Check sheet for the modelled part. Datum: model origin and axes. Units: mm. Face numbers are marked on the shaded views. A direction names the side the tool comes from. Give positions to 0.01 mm unless a question says otherwise; leave off trailing zeros. Order: outer loops, then holes, each group sorted by start corner. A loop starts at its lowest first (then second) coordinate and runs counter-clockwise, first axis right, second up.
Item 1: Sectioned sample at D-D on x = 18.5. Record the boundary of the cut face in (y, z), and give its area (3 significant figures).
Item 2: Material ranges on line 1 along X through (y, z) = (40, -12.5); line 2 along X through (y, z) = (-32, -9.75); line 3 along Y through (x, z) = (-2, -4), recorded low to high.
Item 3: Sectioned sample at A-A on y = -24. Record the boundary of the cut face in (x, z).
Item 4: Gauge pin test, flat ends, axial feed: P1, Ø1.6, axis at y = 19, z = -6, coming from the -X side; P2, Ø1.5, axis at y = 0.5, z = -22, coming from the -X side; P3, Ø0.6, axis at x = 0.5, z = -6, coming from the +Y side. Record the tip position at first contact, or that the pin passes through.
Item 5: Access from +Z, -Z, +X, -X, +Y, -Y to the whole of each face (thin tool, end or side, straight path). Record for the marked faces 5, 6, 7 and 8.
Item 6: Sectioned sample at C-C on y = 35. Record the boundary of the cut face in (x, z), and give its area (3 significant figures).
Item 7: Release check for a two-part mould opening along X. For the marked faces 1, 2, 3 and 4 record: released by +X, released by -X, zero draft, split by the parting line, or undercut.
Item 8: Sectioned sample at B-B on z = -16.5. Count the separate pieces of the cut face and the enclosed holes in it, and give its area (3 significant figures).
from build123d import *

# Parameters (mm, degrees)
CROQUIS1_W              = 20.84578855
CROQUIS1_H              = 73.5
SALIENTE_EXTRUIR1_DEPTH = 30
CROQUIS2_W              = 20.84578855
CROQUIS2_H              = 30
CROQUIS2_W_2            = 18
CROQUIS2_H_2            = 2
SALIENTE_EXTRUIR2_DEPTH = 2
CROQUIS3_W              = 20.84578855
CROQUIS3_H              = 30
CROQUIS3_W_2            = 18.44578855
CROQUIS3_H_2            = 27.6
SALIENTE_EXTRUIR3_DEPTH = 24
CORTAR_EXTRUIR1_DEPTH   = 12
CROQUIS6_W              = 10
CROQUIS6_H              = 2.1
CORTAR_EXTRUIR2_DEPTH   = 12
CROQUIS7_W              = 5
CROQUIS7_H              = 72.3
CORTAR_EXTRUIR3_DEPTH   = 81
REDONDEO1_R             = 2
SALIENTE_EXTRUIR4_DEPTH = 30
CORTAR_EXTRUIR4_DEPTH   = 30
CROQUIS11_W             = 3.5
CROQUIS11_H             = 18.8
CORTAR_EXTRUIR5_DEPTH   = 30
REDONDEO2_R             = 1


with BuildPart() as part:
    # Croquis1 → Saliente-Extruir1 (new body)
    with BuildSketch(Plane.XY):
        with Locations((4.194544399, -18.730645161)):
            Rectangle(CROQUIS1_W, CROQUIS1_H)
    extrude(amount=-SALIENTE_EXTRUIR1_DEPTH)

    # Croquis2 → Saliente-Extruir2 (add)
    with BuildSketch(Plane(origin=(0, 18.019354839, 0), x_dir=(1, 0, 0), z_dir=(0, 1, 0))):
        with Locations((4.194544399, 15)):
            Rectangle(CROQUIS2_W, CROQUIS2_H)
        with Locations((4.194544399, 6)):
            Rectangle(CROQUIS2_W_2, CROQUIS2_H_2, mode=Mode.SUBTRACT)
    extrude(amount=SALIENTE_EXTRUIR2_DEPTH)

    # Croquis3 → Saliente-Extruir3 (add)
    with BuildSketch(Plane(origin=(0, 20.019354839, 0), x_dir=(1, 0, 0), z_dir=(0, 1, 0))):
        with Locations((4.194544399, 15)):
            Rectangle(CROQUIS3_W, CROQUIS3_H)
        with Locations((4.194544399, 15)):
            Rectangle(CROQUIS3_W_2, CROQUIS3_H_2, mode=Mode.SUBTRACT)
    extrude(amount=SALIENTE_EXTRUIR3_DEPTH)

    # Croquis4 → Cortar-Extruir1 (cut)
    with BuildSketch(Plane.XY):
        with BuildLine():
            Line((3.194544399, 33.436155454), (5.194544399, 33.436155454))
            ThreePointArc((5.194544399, 33.436155454), (6.608757961, 32.850369016), (7.194544399, 31.436155454))
            Line((7.194544399, 31.436155454), (7.194544399, 29.436155454))
            ThreePointArc((7.194544399, 29.436155454), (6.608757961, 28.021941892), (5.194544399, 27.436155454))
            Line((5.194544399, 27.436155454), (3.194544399, 27.436155454))
            ThreePointArc((3.194544399, 27.436155454), (1.780330837, 28.021941892), (1.194544399, 29.436155454))
            Line((1.194544399, 29.436155454), (1.194544399, 31.436155454))
            ThreePointArc((1.194544399, 31.436155454), (1.780330837, 32.850369016), (3.194544399, 33.436155454))
        make_face()
    extrude(amount=-CORTAR_EXTRUIR1_DEPTH, mode=Mode.SUBTRACT)

    # Croquis6 → Cortar-Extruir2 (cut)
    with BuildSketch(Plane.XY.offset(-28.8)):
        with Locations((4.194544399, 21.069354839)):
            Rectangle(CROQUIS6_W, CROQUIS6_H)
    extrude(amount=-CORTAR_EXTRUIR2_DEPTH, mode=Mode.SUBTRACT)

    # Croquis7 → Cortar-Extruir3 (cut)
    with BuildSketch(Plane.XY):
        with Locations((-3.728349876, -19.330645161)):
            Rectangle(CROQUIS7_W, CROQUIS7_H)
        with Locations((12.117438674, -19.330645161)):
            Rectangle(CROQUIS7_W, CROQUIS7_H)
    extrude(amount=-CORTAR_EXTRUIR3_DEPTH, mode=Mode.SUBTRACT)

    # Redondeo1
    redondeo1_edges = [part.edges().sort_by_distance(p)[0] for p in [
        (-6.228349876, 16.819354839, -15),
        (-1.228349876, 16.819354839, -15),
        (14.617438674, 16.819354839, -15),
        (9.617438674, 16.819354839, -15),
        (-6.228349876, 30.419354839, -30),
        (14.617438674, 30.419354839, -30),
        (-6.228349876, 30.419354839, 0),
        (14.617438674, 30.419354839, 0),
    ]]
    fillet(redondeo1_edges, radius=REDONDEO1_R)

    # Croquis9 → Saliente-Extruir4 (add)
    with BuildSketch(Plane.XY):
        with BuildLine():
            Line((-20.805455601, -55.480645161), (29.194544399, -55.480645161))
            Line((29.194544399, -55.480645161), (29.194544399, -51.480645161))
            Line((29.194544399, -51.480645161), (19.617438674, -51.480645161))
            ThreePointArc((19.617438674, -51.480645161), (12.546370862, -48.551712973), (9.617438674, -41.480645161))
            Line((9.617438674, -41.480645161), (9.617438674, -20.330645161))
            Line((9.617438674, -20.330645161), (-1.228349876, -20.330645161))
            Line((-1.228349876, -20.330645161), (-1.228349876, -41.480645161))
            ThreePointArc((-1.228349876, -41.480645161), (-4.157282064, -48.551712973), (-11.228349876, -51.480645161))
            Line((-11.228349876, -51.480645161), (-20.805455601, -51.480645161))
            Line((-20.805455601, -51.480645161), (-20.805455601, -55.480645161))
        make_face()
    extrude(amount=-SALIENTE_EXTRUIR4_DEPTH)

    # Croquis10 → Cortar-Extruir4 (cut)
    with BuildSketch(Plane(origin=(0, -51.480645161, 0), x_dir=(1, 0, 0), z_dir=(0, 1, 0))):
        with BuildLine():
            Line((25.824740978, 25), (25.824740978, 5))
            ThreePointArc((25.824740978, 5), (23.724740978, 2.9), (21.624740978, 5))
            Line((21.624740978, 5), (21.624740978, 25))
            ThreePointArc((21.624740978, 25), (23.724740978, 27.1), (25.824740978, 25))
        make_face()
        with BuildLine():
            Line((-17.43565218, 25), (-17.43565218, 5))
            ThreePointArc((-17.43565218, 5), (-15.33565218, 2.9), (-13.23565218, 5))
            Line((-13.23565218, 5), (-13.23565218, 25))
            ThreePointArc((-13.23565218, 25), (-15.33565218, 27.1), (-17.43565218, 25))
        make_face()
    extrude(amount=-CORTAR_EXTRUIR4_DEPTH, mode=Mode.SUBTRACT)

    # Croquis11 → Cortar-Extruir5 (cut)
    with BuildSketch(Plane.XY):
        with Locations((4.194544399, 6.119354839)):
            Rectangle(CROQUIS11_W, CROQUIS11_H)
        with Locations((4.194544399, -16.680645161)):
            Rectangle(CROQUIS11_W, CROQUIS11_H)
        with Locations((4.194544399, -39.480645161)):
            Rectangle(CROQUIS11_W, CROQUIS11_H)
    extrude(amount=-CORTAR_EXTRUIR5_DEPTH, mode=Mode.SUBTRACT)

    # Redondeo2
    redondeo2_edges = [part.edges().sort_by_distance(p)[0] for p in [
        (2.444544399, -3.280645161, -15),
        (2.444544399, 15.519354839, -15),
        (5.944544399, 15.519354839, -15),
        (5.944544399, -3.280645161, -15),
        (2.444544399, -26.080645161, -15),
        (2.444544399, -7.280645161, -15),
        (5.944544399, -7.280645161, -15),
        (5.944544399, -26.080645161, -15),
        (2.444544399, -48.880645161, -15),
        (2.444544399, -30.080645161, -15),
        (5.944544399, -30.080645161, -15),
        (5.944544399, -48.880645161, -15),
    ]]
    fillet(redondeo2_edges, radius=REDONDEO2_R)


solid = part.part
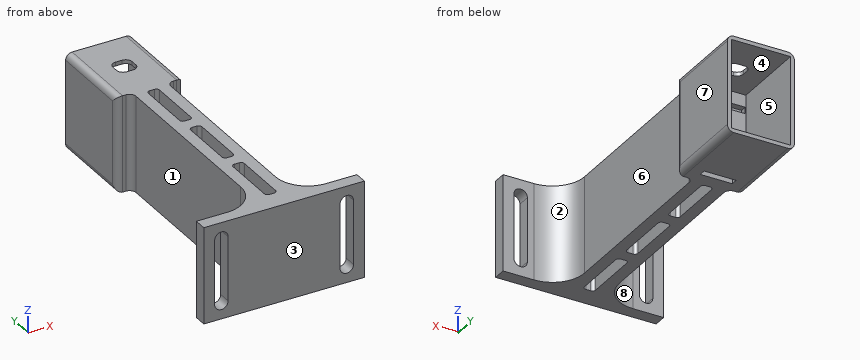
Report:
1. outline: (-55.48, -30) - (-51.42, -30) - (-51.42, 0) - (-55.48, 0) - close
1. area: 122 mm2
2. line 1: x = -6.23 to -5.03, 13.42 to 14.62
2. line 2: x = -1.23 to 2.44, 5.94 to 9.62
2. line 3: y = -55.48 to -45.33, 16.4 to 20.02
3. outline: (-1.23, -30) - (2.44, -30) - (2.44, 0) - (-1.23, 0) - close; (5.94, -30) - (9.62, -30) - (9.62, 0) - (5.94, 0) - close
4. P1: stops at x = -6.23
4. P2: stops at x = -1.23
4. P3: stops at y = 18.02
5. face 5: +Y
5. face 6: +Z, -Z, +X
5. face 7: +Z, -Z, +X, +Y
5. face 8: +Z, -Z, -X
6. outline: (-6.23, -28) arc R2 ccw to (-4.23, -30) - (12.62, -30) arc R2 ccw to (14.62, -28) - (14.62, -2) arc R2 ccw to (12.62, 0) - (-4.23, 0) arc R2 ccw to (-6.23, -2) - close; hole (-5.03, -28.8) - (13.42, -28.8) - (13.42, -1.2) - (-5.03, -1.2) - close
6. area: 113 mm2
7. face 1: released by -X
7. face 2: released by +X
7. face 3: zero draft
7. face 4: undercut
8. separate pieces: 3
8. enclosed holes: 3
8. area: 880 mm2
